Part model, mm, in its own coordinate system. A direction names the side the tool comes from. Round coordinates to 2 decimals unless told otherwise and drop trailing zeros. Order: outer loops, then holes, each group sorted by start corner. A loop starts at its lowest first (then second) coordinate and runs counter-clockwise, first axis right, second up. Notation, with made-up numbers: M -25,0.5 L -16,0.5 A8 cw -16,12.5 Z; hole C 46.25,28 d4. An arc over 180 degrees is marked long. One line per question, with ' | ' between items.
Autodesk Fusion 360 part; units mm, degrees
sketch "Skizze1" plane through (0, 0, 0) normal (0, 0, 1) x (1, 0, 0)
  line L0 (30, 20) -> (-30, 20)
  line L1 (-30, 20) -> (-30, -20)
  line L2 (-30, -20) -> (30, -20)
  line L3 (30, -20) -> (30, 20)
  line L4 (30, 20) -> (-30, -20) construction
  line L5 (-30, 20) -> (30, -20) construction
  dimension "d2" = 60
  dimension "d3" = 40
extrude "Extrusion1" add sketch "Skizze1" along normal blind 195 makes body 1
sketch "Skizze3" plane through (0, -20, 0) normal (0, -1, 0) x (1, 0, 0)
  line L0 (-30, 0) -> (30, 0)
  line L1 (30, 0) -> (30, 195)
  line L2 (30, 195) -> (-30, 195)
  line L3 (-30, 195) -> (-30, 0)
  line L4 (3.1, 8.1) -> (3.1, 56.9)
  arc A0 (3.1, 56.9) -> (-3.1, 56.9) centre (0, 56.9) ccw
  line L5 (-3.1, 56.9) -> (-3.1, 8.1)
  arc A1 (-3.1, 8.1) -> (3.1, 8.1) centre (0, 8.1) ccw
  line L6 (0, 5) -> (0, 60) construction
  line L7 (2.5, 72.5) -> (2.5, 97.5)
  arc A2 (2.5, 97.5) -> (-2.5, 97.5) centre (0, 97.5) ccw
  line L8 (-2.5, 97.5) -> (-2.5, 72.5)
  arc A3 (-2.5, 72.5) -> (2.5, 72.5) centre (0, 72.5) ccw
  line L9 (0, 70) -> (0, 100) construction
  point P0 (0, 195)
  dimension "d20" = 6.2
  dimension "d21" = 5
extrude "Extrusion2" cut sketch "Skizze3" against normal blind 40 contours L4 A0 L5 A1 | L7 A2 L8 A3 bodies 1
sketch "Skizze4" plane through (30, 0, 0) normal (1, 0, 0) x (0, 1, 0)
  line L0 (-20, 0) -> (20, 0)
  line L1 (20, 0) -> (20, 195)
  line L2 (20, 195) -> (-20, 195)
  line L3 (-20, 195) -> (-20, 0)
  circle A0 centre (0, 174.5) radius 4.15
  dimension "d12" = 8.3
extrude "Extrusion3" add sketch "Skizze4" against normal blind 60 separate body contours A0 makes body 2
sketch "Skizze6" plane through (0, 0, 0) normal (0, 1, 0) x (1, 0, 0)
sketch "Skizze7" plane through (0, 20, 0) normal (0, 1, 0) x (-1, 0, 0)
  line L0 (-30, 0) -> (30, 0)
  line L1 (30, 0) -> (30, 195)
  line L2 (30, 195) -> (-30, 195)
  line L3 (-30, 195) -> (-30, 0)
  circle A0 centre (0, 160) radius 2.5
  line L4 (-2.5, 72.5) -> (-2.5, 97.5)
  arc A1 (2.5, 97.5) -> (-2.5, 97.5) centre (0, 97.5) ccw
  line L5 (2.5, 97.5) -> (2.5, 72.5)
  arc A2 (-2.5, 72.5) -> (2.5, 72.5) centre (0, 72.5) ccw
  line L6 (-3.1, 8.1) -> (-3.1, 56.9)
  arc A3 (3.1, 56.9) -> (-3.1, 56.9) centre (0, 56.9) ccw
  line L7 (3.1, 56.9) -> (3.1, 8.1)
  arc A4 (-3.1, 8.1) -> (3.1, 8.1) centre (0, 8.1) ccw
  dimension "d17" = 5
extrude "Extrusion4" cut sketch "Skizze7" against normal blind 40 contours A0 bodies 1
sketch "Skizze8" plane through (0, -20, 0) normal (0, -1, 0) x (1, 0, 0)
  circle A0 centre (0, 160) radius 2.5
  line L0 (2.5, 97.5) -> (2.5, 72.5)
  arc A1 (-2.5, 72.5) -> (2.5, 72.5) centre (0, 72.5) ccw
  line L1 (-2.5, 72.5) -> (-2.5, 97.5)
  arc A2 (2.5, 97.5) -> (-2.5, 97.5) centre (0, 97.5) ccw
  line L2 (3.1, 56.9) -> (3.1, 8.1)
  arc A3 (-3.1, 8.1) -> (3.1, 8.1) centre (0, 8.1) ccw
  line L3 (-3.1, 8.1) -> (-3.1, 56.9)
  arc A4 (3.1, 56.9) -> (-3.1, 56.9) centre (0, 56.9) ccw
  line L4 (-30, 0) -> (30, 0)
  line L5 (30, 0) -> (30, 195)
  line L6 (30, 195) -> (-30, 195)
  line L7 (-30, 195) -> (-30, 0)
  line L8 (5, 72) -> (5, 98)
  arc A5 (5, 98) -> (-5, 98) centre (0, 98) ccw
  line L9 (-5, 98) -> (-5, 72)
  arc A6 (-5, 72) -> (5, 72) centre (0, 72) ccw
  line L10 (0, 72) -> (0, 98) construction
extrude "Extrusion5" cut sketch "Skizze8" against normal blind 9 contours L8 A5 L9 A6 bodies 1
extrude "Extrusion7" cut 1 faces at (-30, -1.0141, 173.1467) along direction (1, 0, 0) blind 50 on bodies 2 bodies 1 2
combine "Kombinieren2" operation add target body 1 tool bodies 2
1) Which spindle directions (+Z, -Z, +X, -X, +Y, -Y) get a long thin tool onto all of the face, cutting with end or side? Do faces 4 (the face through (0, 0, 0)), 5 (the face through (-5.35, -0.9, 178.55)), 6 (the face through (-3.1, 0, 33)), 7 (the face through (0, -16, 103)). Say none if no direction does.
The answers:
face 4: -Z, +X, -X, +Y, -Y | face 5: -X | face 6: +Y, -Y | face 7: -Y
2) Saw through at C-C (x = 0). List the corners of the cut face in (y, z).
The answers:
outline: M -20,0 L 20,0 L 20,5 L -20,5 Z; M -20,60 L 20,60 L 20,70 L -11,70 L -11,67 L -20,67 Z; M -20,103 L -11,103 L -11,100 L 20,100 L 20,157.5 L -20,157.5 Z; M -20,162.5 L 20,162.5 L 20,195 L -20,195 Z; hole C 0,174.5 d8.3
3) Drop a flat-ended pin along its axis: pin 1 (2.5 mm diameter, centred on y = -1, z = 173.5, fed in from -X). Give the stop position or say it passes through.
The answers:
pin 1: stops at x = 20
4) Two-plate mould, pull along Z, no slides. Class faces 1 (the face through (0, 4, 70)), 2 (the face through (7, 20, 96)), 3 (the face through (0, 0, 195)): released by +Z, released by -Z, zero draft, split by the parting line, or undercut.
The answers:
face 1: undercut | face 2: zero draft | face 3: released by +Z
5) Saw through at A-A (z = 52.5). List the corners of the cut face in (x, y).
The answers:
outline: M -30,-20 L -3.1,-20 L -3.1,20 L -30,20 Z; M 3.1,-20 L 30,-20 L 30,20 L 3.1,20 Z
6) Saw through at B-B (y = -7). List the corners of the cut face in (x, z), plus the area to 3 significant figures.
The answers:
outline: M -30,0 L 30,0 L 30,195 L -30,195 Z; hole M -3.1,8.1 A3.1 ccw 3.1,8.1 L 3.1,56.9 A3.1 ccw -3.1,56.9 Z; hole M -2.5,72.5 A2.5 ccw 2.5,72.5 L 2.5,97.5 A2.5 ccw -2.5,97.5 Z; hole C 0,160 d5 | area: 11,200 mm²
7) Saw through at D-D (y = -16.5). List the corners of the cut face in (x, z), plus the area to 3 significant figures.
The answers:
outline: M -30,0 L 30,0 L 30,195 L -30,195 Z; hole M -5,72 A5 ccw 5,72 L 5,98 A5 ccw -5,98 Z; hole M -3.1,8.1 A3.1 ccw 3.1,8.1 L 3.1,56.9 A3.1 ccw -3.1,56.9 Z; hole C 0,160 d5 | area: 11,000 mm²
8) Probe line 1 (Z direction, x = 0, y = -9); line 2 (X direction, y = -15, z = 91); line 3 (Y direction, x = -13, z = 174). List the from-to ranges inside material, lowest first. Write a range as [from, to].
The answers:
line 1: z = [0, 5], [60, 70], [100, 157.5], [162.5, 195] | line 2: x = [-30, -5], [5, 30] | line 3: y = [-20, -4.12], [4.12, 20]
